from build123d import *

# Parameters (mm, degrees)
SKETCH_1_W      = 25
SKETCH_1_H      = 30
EXTRUDE_1_DEPTH = 1.6
SKETCH_2_R      = 9.6
EXTRUDE_2_DEPTH = 58.9
SKETCH_4_R      = 5.65
EXTRUDE_3_DEPTH = 9.5


with BuildPart() as part:
    # ｽｹｯﾁ1 → ﾎﾞｽ - 押し出し1 (new body)
    with BuildSketch(Plane.XY):
        with Locations((-14.765846009, 19.364285714)):
            Rectangle(SKETCH_1_W, SKETCH_1_H)
    extrude(amount=EXTRUDE_1_DEPTH)

    # ｽｹｯﾁ2 → ﾎﾞｽ - 押し出し2 (add)
    with BuildSketch(Plane.XY.offset(1.6)):
        with Locations(Location((-14.765846009, 21.864285714, 0), (0, 0, 180))):
            Circle(SKETCH_2_R)
    extrude(amount=EXTRUDE_2_DEPTH)

    # ｽｹｯﾁ4 → ﾎﾞｽ - 押し出し3 (add)
    with BuildSketch(Plane.XY.offset(60.5)):
        with Locations((-14.765846009, 21.864285714)):
            Circle(SKETCH_4_R)
    extrude(amount=EXTRUDE_3_DEPTH)


solid = part.part
Input: part model. Units: mm. Frame: model coordinates. A direction names the side the tool comes from. Round coordinates to 2 decimals unless told otherwise and drop trailing zeros. Order: outer loops, then holes, each group sorted by start corner. A loop starts at its lowest first (then second) coordinate and runs counter-clockwise, first axis right, second up. Notation, with made-up numbers: (-1.5, 86.5) - (24.5, 86.5) arc R26 ccw to (24.5, 113.5) - close; hole circle Ø2 at (-9.5, 69). An arc over 180 degrees is marked (long way). Answer as a JSON object with one key per item and string values. Group by question number.
(1) Cut plane B-B (x = -11). Return loops of the section in (y, z).
(2) Material intervals for probe 1 along Z at (x, y) = (-22, 11); probe 2 along Z at (x, y) = (-22.5, 25); probe 3 along Y at (x, z) = (-14.5, 9.5), sorted ascending. Write a range as from..to.
(3) Cut plane C-C (z = 32.5). Return loops of the section in (x, y), then the cut area to 3 significant figures.
(4) Reachability of faces 1 (the face through (-2.266, 19, 1)), 2 (the face through (-20, 13, 1.6)) from +Z, -Z, +X, -X, +Y, -Y: full face, straight path, thin tool, end or side. Return the list, or none.
(5) Pin query (flat end, axial travel): P1, Ø5, axis at y = 18, z = 21, coming from the +X side; P2, Ø6, axis at x = -15.5, y = 8.5, coming from the +Z side; P3, Ø12, axis at x = -22.5, z = 12, coming from the +Y side; P4, Ø2, axis at x = -16, y = 31, coming from the -Z side. Return the tip coordinate at first contact, or that it passes through.
(6) Cut plane D-D (x = -18.5). Return loops of the section in (y, z).
(7) Cut plane A-A (y = 13). Return loops of the section in (x, z).
Here are the results:
{
 "1": {"outline": "(4.36, 0) - (34.36, 0) - (34.36, 1.6) - (30.69, 1.6) - (30.69, 60.5) - (26.08, 60.5) - (26.08, 70) - (17.65, 70) - (17.65, 60.5) - (13.03, 60.5) - (13.03, 1.6) - (4.36, 1.6) - close"},
 "2": {"probe 1": "z = 0..1.6", "probe 2": "z = 0..60.5", "probe 3": "y = 12.27..31.46"},
 "3": {"outline": "circle Ø19.2 at (-14.77, 21.86)", "area": "290 mm^2"},
 "4": {"face 1": "+Z, -Z, +X, +Y, -Y", "face 2": "+Z"},
 "5": {"P1": "stops at x = -5.26", "P2": "stops at z = 1.6", "P3": "stops at y = 31.31", "P4": "stops at z = 0"},
 "6": {"outline": "(4.36, 0) - (34.36, 0) - (34.36, 1.6) - (30.71, 1.6) - (30.71, 60.5) - (26.1, 60.5) - (26.1, 70) - (17.62, 70) - (17.62, 60.5) - (13.02, 60.5) - (13.02, 1.6) - (4.36, 1.6) - close"},
 "7": {"outline": "(-27.27, 0) - (-2.27, 0) - (-2.27, 1.6) - (-11.08, 1.6) - (-11.08, 60.5) - (-18.45, 60.5) - (-18.45, 1.6) - (-27.27, 1.6) - close"}
}
